from build123d import *

# Parameters (mm, degrees)
F1_DEPTH       = 12
F2_D           = 5.5
F2_CBORE_D     = 9.75
F2_CBORE_DEPTH = 5
F3_R           = 4.99999


# Not quite as in the source:
# - a fillet or chamfer is up to 0.001 mm smaller than in the source, because OpenCascade refuses the exact size


with BuildPart() as f1:
    # F0 (on Top) → F1 (new body)
    with BuildSketch(Plane.XY):
        with BuildLine():
            Line((80, 10), (0, 10))
            ThreePointArc((0, 10), (-7.0710678119, 7.0710678119), (-10, 0))
            Line((-10, 0), (-10, -40))
            ThreePointArc((-10, -40), (-5.2573111212, -48.5065080835), (4.472135955, -48.94427191))
            Line((4.472135955, -48.94427191), (84.472135955, -8.94427191))
            ThreePointArc((84.472135955, -8.94427191), (89.7324898947, 2.2975292055), (80, 10))
        make_face()
        with BuildLine():
            ThreePointArc((51.527864045, -10), (53.4743620239, -11.5404941589), (52.422291236, -13.788854382))
            Line((52.422291236, -13.788854382), (12.894427191, -33.5527864045))
            ThreePointArc((12.894427191, -33.5527864045), (10.9485377758, -33.4652336392), (10, -31.7639320225))
            Line((10, -31.7639320225), (10, -12))
            ThreePointArc((10, -12), (10.5857864376, -10.5857864376), (12, -10))
            Line((12, -10), (51.527864045, -10))
        make_face(mode=Mode.SUBTRACT)
    extrude(amount=F1_DEPTH)

    # F2 (through all)
    with Locations(Plane(origin=(0, 0, 0), x_dir=(1, 0, 0), z_dir=(0, 0, -1))):
        with Locations((80, 0), (0, 40), (40, 0), (0, 15)):
            CounterBoreHole(F2_D / 2, F2_CBORE_D / 2, F2_CBORE_DEPTH)

    # F3 (radius 5 in the source; OpenCascade refuses exactly that, so slightly less here)
    f3_edges = [f1.edges().sort_by_distance(p)[0] for p in [
        (44.472136, -28.944272, 0),
        (31.763932, -10, 0),
    ]]
    fillet(f3_edges, radius=F3_R)


solid = f1.part
Build history of the part. All positions in model axes, mm. A direction names the side the tool comes from. Coordinates: 2 decimals unless noted, no trailing zeros. Order: outer loops, then holes, each group sorted by start corner. A loop starts at its lowest first (then second) coordinate and runs counter-clockwise, first axis right, second up. Notation, with made-up numbers: (22.25, -3.5) -> (76.25, -3.5) arc R15 ccw to (76.25, 0.5) -> close; hole circle Ø3 at (44.5, -3.75). An arc over 180 degrees is marked (long way). One line per item, written item: value.
(1) Slice it at C-C, the plane z = 1.75. List the corners of the cut face in (x, y) (3 decimals), plus the area to 3 significant figures.
Checked values:
outline: (-8.8, -40) arc R8.8 ccw to (3.935, -47.871) -> (83.935, -7.871) arc R8.8 ccw to (80, 8.8) -> (0, 8.8) arc R8.8 ccw to (-8.8, 0) -> close; hole circle Ø9.75 at (0, -40); hole circle Ø9.75 at (0, -15); hole (8.8, -31.764) arc R3.2 ccw to (13.431, -34.626) -> (52.959, -14.862) arc R3.2 ccw to (51.528, -8.8) -> (12, -8.8) arc R3.2 ccw to (8.8, -12) -> close; hole circle Ø9.75 at (40, 0); hole circle Ø9.75 at (80, 0)
area: 2,630 mm2
(2) Mould opens along Y. For faces 4 (the flat face through (-10, -20, 8)), 5 (the cylindrical face through (44.65, -1.46, 2.46)), 6 (the cylindrical face through (33.05, -25.15, 1.43)), 7 (the flat face through (41, 10, 8)) say: pulls with the +Y half, pulls with the -Y half, needs draft (parallel to the pull), parting line crosses it, or undercut.
Checked values:
face 4: needs draft
face 5: undercut
face 6: undercut
face 7: pulls with the +Y half
(3) Probe line 1 (Y direction, x = 0, z = 10.5); line 2 (X direction, y = -15.5, z = 6.75); line 3 (Y direction, x = 2, z = 9). List the from-to ranges inside material, lowest first. Write a range as [from, to].
Checked values:
line 1: [-50, -42.75], [-37.25, -17.75], [-12.25, 10]
line 2: [-10, -2.7], [2.7, 10], [49, 71.36]
line 3: [-49.8, -41.89], [-38.11, -16.89], [-13.11, 10]
(4) Slice it at A-A, the plane z = 8.25. List the corners of the cut face in (x, y).
Checked values:
outline: (-10, -40) arc R10 ccw to (4.47, -48.94) -> (84.47, -8.94) arc R10 ccw to (80, 10) -> (0, 10) arc R10 ccw to (-10, 0) -> close; hole circle Ø5.5 at (0, -40); hole circle Ø5.5 at (0, -15); hole (10, -31.76) arc R2 ccw to (12.89, -33.55) -> (52.42, -13.79) arc R2 ccw to (51.53, -10) -> (12, -10) arc R2 ccw to (10, -12) -> close; hole circle Ø5.5 at (40, 0); hole circle Ø5.5 at (80, 0)
(5) Drop flat-ended pins along their axis: pin 1 Ø1 at (x, z) = (67, 8) entering from -Y; pin 2 Ø1 at (x, y) = (8, -43.5) entering from -Z; pin 3 Ø6 at (x, y) = (0, -15) entering from -Z; pin 4 Ø3.5 at (x, y) = (0, -15) entering from +Z. Give the stop position or say it passes through.
Checked values:
pin 1: y = -17.93
pin 2: z = 0.15
pin 3: z = 5
pin 4: through
(6) Slice it at B-B, the plane x = 40. Count the separate pieces of the cut face and the enclosed holes in it, plus the area to 3 significant figures.
Checked values:
separate pieces: 3
enclosed holes: 0
area: 264 mm2
(7) Tool access for faces 1 (the cylindrical face through (53.465, -11.504, 8.451)), 2 (the cylindrical face through (89.774, 2.115, 8.451)), 3 (the cylindrical face through (-0.635, -44.834, 2.465)): list every direction of +Z, -Z, +X, -X, +Y, -Y with a clear straight run to the whole face (end or side of a thin tool).
Checked values:
face 1: +Z, -Z
face 2: +Z, -Z, +X
face 3: -Z
